Input: part model. Units: mm. Frame: model coordinates. Give positions to 0.01 mm unless a question says otherwise; leave off trailing zeros. Loops run counter-clockwise (first coordinate to the right, second up) from the corner with the lowest first, then second, coordinate; pieces in that order, holes last. Notation, with made-up numbers: M -26,-27.5 L -8,-27.5 A20 cw -8,-13.5 Z; hole C -36.75,28.25 d6. An arc over 180 degrees is marked long. One line per item, written item: value. Start each with the question number.
(1) Section C-C on x = -15. Output: boundary loops of the cut face in (y, z).
(2) Section D-D on z = -10.5. Output: boundary loops of the cut face in (x, y), plus the area to 3 significant figures.
(3) Section A-A on z = 25. Output: boundary loops of the cut face in (x, y), plus the area to 3 significant figures.
(4) Section B-B on y = -0.4. Output: boundary loops of the cut face in (x, z), plus the area to 3 significant figures.
(5) Ray query, line 1 along X through (y, z) = (1.5, 25); line 2 along Y through (x, z) = (-7, -9.5); line 3 along X through (y, z) = (-1.65, 32). Return the intervals inside material, ascending. Write a range as from..to.
(6) Pin query (flat end, axial travel): P1, Ø4, axis at x = 0, z = 25, coming from the +Y side; P2, Ø1.5, axis at x = 15, y = -1, coming from the -Z side; P3, Ø2, axis at x = -6.5, y = -1, coming from the +Z side; P4, Ø1, axis at y = 0, z = 53.5, coming from the -X side. Return the tip coordinate at first contact, or that it passes through.
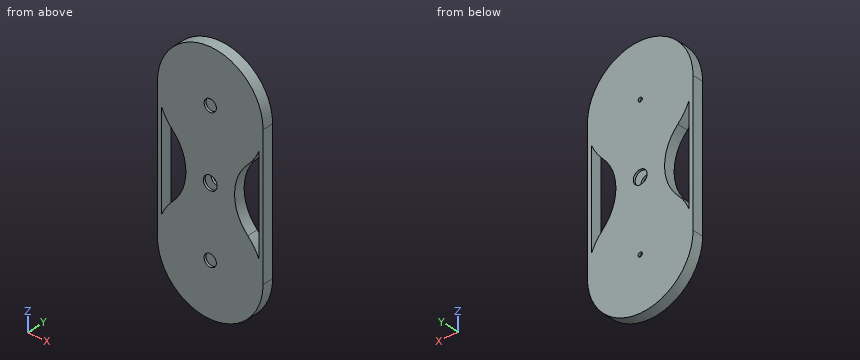
```python
from build123d import *

# Parameters (mm, degrees)
BOSS_EXTRUDE1_DEPTH      = 2
BOSS_EXTRUDE1_DEPTH_BACK = 2
CUT_EXTRUDE1_DEPTH       = 1.2
CUT_EXTRUDE1_DEPTH_BACK  = 1.2
SKETCH4_W                = 7
SKETCH4_H                = 11
BOSS_EXTRUDE2_DEPTH      = 1.2
SWEEP1_PROFILE_R         = 1
SKETCH25_R               = 2.2
CUT_EXTRUDE2_DEPTH       = 2.2
SKETCH26_R               = 2.5
SKETCH26_R_2             = 0.75
CUT_EXTRUDE3_DEPTH       = 10.2
CUT_EXTRUDE4_DEPTH       = 10
CUT_EXTRUDE4_DEPTH_BACK  = 10


with BuildPart() as part:
    # Sketch1 → Boss-Extrude1 (new body, two sides)
    with BuildSketch(Plane(origin=(0, 0, 0), x_dir=(1, 0, 0), z_dir=(0, 1, 0))) as boss_extrude1_sk:
        with BuildLine():
            Line((-19, 0), (-19, -50))
            ThreePointArc((-19, -50), (0, -69), (19, -50))
            Line((19, -50), (19, 0))
            ThreePointArc((19, 0), (0, 19), (-19, 0))
        make_face()
    extrude(amount=BOSS_EXTRUDE1_DEPTH)
    extrude(boss_extrude1_sk.sketch, amount=-BOSS_EXTRUDE1_DEPTH_BACK)

    # Sketch3 → Cut-Extrude1 (cut, two sides)
    with BuildSketch(Plane(origin=(0, 0, 0), x_dir=(1, 0, 0), z_dir=(0, 1, 0))) as cut_extrude1_sk:
        with BuildLine():
            ThreePointArc((12.445079349, -12.445079349), (7.244660941, -25), (12.445079349, -37.554920651))
            ThreePointArc((12.445079349, -37.554920651), (0, -67.6), (-12.445079349, -37.554920651))
            ThreePointArc((-12.445079349, -37.554920651), (-7.244660941, -25), (-12.445079349, -12.445079349))
            ThreePointArc((-12.445079349, -12.445079349), (0, 17.6), (12.445079349, -12.445079349))
        make_face()
    extrude(amount=CUT_EXTRUDE1_DEPTH, mode=Mode.SUBTRACT)
    extrude(cut_extrude1_sk.sketch, amount=-CUT_EXTRUDE1_DEPTH_BACK, mode=Mode.SUBTRACT)

    # Sketch4 → Boss-Extrude2 (add)
    with BuildSketch(Plane.XZ.offset(2)):
        with Locations((-13.5, 25)):
            Rectangle(SKETCH4_W, SKETCH4_H)
        with Locations((13.5, 25)):
            Rectangle(SKETCH4_W, SKETCH4_H)
    extrude(amount=BOSS_EXTRUDE2_DEPTH)

    # Sweep1: sweep along a path in Sketch6
    with BuildLine(Plane(origin=(-13.5, 0, 0), x_dir=(0, 0, -1), z_dir=(1, 0, 0))) as sweep1_path:
        Line((-22.3, -3.2), (-22.3, -5.3))
        ThreePointArc((-22.3, -5.3), (-24.369122081, -7.65570217), (-26.972043675, -5.907732468))
    # Sweep1 profile (on start of the path) → Sweep1 (sweep)
    with BuildSketch(Plane(origin=(-13.5, -3.2, 22.3), x_dir=(0, 0, -1), z_dir=(0, -1, 0))):
        Circle(SWEEP1_PROFILE_R)
    sweep1 = sweep(path=sweep1_path.line)

    # Mirror1: Sweep1 across plane
    add(sweep1.mirror(Plane(origin=(0, 0, 0), x_dir=(0, 0, 1), z_dir=(1, 0, 0))))

    # Sketch25 → Cut-Extrude2 (cut)
    with BuildSketch(Plane.XZ.offset(2)):
        Circle(SKETCH25_R)
        with Locations((0, 50)):
            Circle(SKETCH25_R)
    extrude(amount=-CUT_EXTRUDE2_DEPTH, mode=Mode.SUBTRACT)

    # Sketch26 → Cut-Extrude3 (cut)
    with BuildSketch(Plane(origin=(0, -2, 0), x_dir=(-1, 0, 0), z_dir=(0, -1, 0))):
        with Locations((0, -25)):
            Circle(SKETCH26_R)
        with Locations((0, -50)):
            Circle(SKETCH26_R_2)
        Circle(SKETCH26_R_2)
    extrude(amount=-CUT_EXTRUDE3_DEPTH, mode=Mode.SUBTRACT)

    # Sketch27 → Cut-Extrude4 (cut, two sides)
    with BuildSketch(Plane.XZ.offset(2)) as cut_extrude4_sk:
        with BuildLine():
            Line((-17.6, 7.419568721), (-17.6, 42.580431279))
            ThreePointArc((-17.6, 42.580431279), (-15.847779861, 39.33895533), (-13.505739521, 36.494260479))
            ThreePointArc((-13.505739521, 36.494260479), (-8.744660941, 25), (-13.505739521, 13.505739521))
            ThreePointArc((-13.505739521, 13.505739521), (-15.847779861, 10.66104467), (-17.6, 7.419568721))
        make_face()
        with BuildLine():
            Line((17.6, 42.580431279), (17.6, 7.419568721))
            ThreePointArc((17.6, 7.419568721), (15.847779861, 10.66104467), (13.505739521, 13.505739521))
            ThreePointArc((13.505739521, 13.505739521), (8.744660941, 25), (13.505739521, 36.494260479))
            ThreePointArc((13.505739521, 36.494260479), (15.847779861, 39.33895533), (17.6, 42.580431279))
        make_face()
    extrude(amount=CUT_EXTRUDE4_DEPTH, mode=Mode.SUBTRACT)
    extrude(cut_extrude4_sk.sketch, amount=-CUT_EXTRUDE4_DEPTH_BACK, mode=Mode.SUBTRACT)


solid = part.part
```
Output values:
1. outline: M -2,-11.66 L 2,-11.66 L 2,11.82 L -2,11.82 Z; M -2,38.18 L 2,38.18 L 2,61.66 L -2,61.66 Z; hole M -1.2,-9.21 L 1.2,-9.21 L 1.2,9.21 L -1.2,9.21 Z; hole M -1.2,40.79 L 1.2,40.79 L 1.2,59.21 L -1.2,59.21 Z
2. outline: M -15.84,-2 L 15.84,-2 L 15.84,2 L -15.84,2 Z; hole M -14.12,-1.2 L 14.12,-1.2 L 14.12,1.2 L -14.12,1.2 Z
2. area: 58.9 mm²
3. outline: M -19,-2 L -17.6,-2 L -17.6,2 L -19,2 Z; M -8.74,-2 L -2.5,-2 L -2.5,-1.2 L -7.24,-1.2 L -7.24,1.2 L -2.5,1.2 L -2.5,2 L -8.74,2 Z; M 2.5,-2 L 8.74,-2 L 8.74,2 L 2.5,2 L 2.5,1.2 L 7.24,1.2 L 7.24,-1.2 L 2.5,-1.2 Z; M 17.6,-2 L 19,-2 L 19,2 L 17.6,2 Z
3. area: 38.4 mm²
4. outline: M -19,0 A19 ccw 19,0 L 19,50 A19 ccw -19,50 Z; hole M -17.6,7.42 A19.1 cw -13.51,13.51 A16.26 ccw -13.51,36.49 A19.1 cw -17.6,42.58 Z; hole M -12.45,12.45 A17.6 ccw long 12.45,12.45 A17.76 cw 12.45,37.55 A17.6 ccw long -12.45,37.55 A17.76 cw Z; hole M 13.51,13.51 A19.1 cw 17.6,7.42 L 17.6,42.58 A19.1 cw 13.51,36.49 A16.26 ccw Z
4. area: 438 mm²
5. line 1: x = -19..-17.6, -8.74..-2.5, 2.5..8.74, 17.6..19
5. line 2: y = -2..-1.2, 1.2..2
5. line 3: x = -19..-17.6, -10.33..10.33, 17.6..19
6. P1: passes through
6. P2: stops at z = -12.57
6. P3: stops at z = 68.19
6. P4: stops at x = -18.76
